Design review of the part built by this model. Coordinates are the model's own, in mm. Face numbers are marked on the shaded views. A direction names the side the tool comes from. Give positions to 0.01 mm unless a question says otherwise; leave off trailing zeros. Loops run counter-clockwise (first coordinate to the right, second up) from the corner with the lowest first, then second, coordinate; pieces in that order, holes last. Notation, with made-up numbers: (36.25, -8.75) -> (46.25, -8.75) arc R34 cw to (46.25, 22.25) -> close; hole circle Ø2 at (-34.5, 31.25). An arc over 180 degrees is marked (long way). Answer in a Markdown table with one row per item. Add a question column.
(1) Draft analysis for pull direction Z (two halves, no side actions). For the marked faces 1, 2 and 3, state which applies: +Z half, -Z half, draft (parallel to the pull), parting line (faces both ways), or undercut.
(2) Consider section A-A on y = 23.5. Write out the cut boundary in (x, z).
(3) Consider section C-C on x = 81. Write out the cut boundary in (y, z).
(4) For the marked faces 4, 5, 6 and 7, list the 3-axis set-ups (+Z, -Z, +X, -X, +Y, -Y) from which the entire face can be reached by the end or side of a thin tool; tool diameter is ignored.
(5) Consider section D-D on y = -4. Count the separate pieces of the cut face and the enclosed holes in it, then the cut area to 3 significant figures.
(6) For line 1 (Z direction, x = 46, y = 7.5); line 2 (X direction, y = 10.5, z = 29); line 3 (Z direction, x = 17, y = 26), list the stretches that pass through material, from the lowest coordinate up.
(7) Consider section B-B on x = 42. Write out the cut boundary in (y, z), then the cut area to 3 significant figures.
(8) For pin 1 (4.5 mm diameter, centred on x = 47, z = 26.5, fed in from +Y); pin 2 (5 mm diameter, centred on x = 32.5, z = 31.5, fed in from +Y); pin 3 (3.5 mm diameter, centred on y = -8.5, z = 35.5, fed in from +X), all flat-tipped, find the tip position at first contact; note any pin that passes through.
from build123d import *

# Parameters (mm, degrees)
BOSS_EXTRU_1_DEPTH       = 84
ESQUISSE6_W              = 27
ESQUISSE6_H              = 47
BOSS_EXTRU_3_DEPTH       = 17
ESQUISSE7_W              = 23.3
ESQUISSE7_H              = 14.3
ENL_V_MAT_EXTRU_4_DEPTH  = 43.3
ESQUISSE8_R              = 1.85
BOSS_EXTRU_4_DEPTH       = 3.5
ESQUISSE12_R             = 11.25
ENL_V_MAT_EXTRU_7_DEPTH  = 2.75
ESQUISSE13_W             = 27
ESQUISSE13_H             = 10
BOSS_EXTRU_5_DEPTH       = 15
ESQUISSE15_W             = 27
ESQUISSE15_H             = 15
ENL_V_MAT_EXTRU_9_DEPTH  = 4
ESQUISSE14_R             = 1.11
ENL_V_MAT_EXTRU_8_DEPTH  = 15
CONG_6_R                 = 5
CONG_7_R                 = 5
CONG_1_R                 = 10
CONG_2_R                 = 10
CONG_3_R                 = 10
CONG_4_R                 = 5
CONG_8_R                 = 5
BOSS_EXTRU_6_DEPTH       = 7.5
ESQUISSE17_R             = 2.25
ENL_V_MAT_EXTRU_10_DEPTH = 110.832109883
ESQUISSE20_W             = 91
ESQUISSE20_H             = 72.5
BOSS_EXTRU_7_DEPTH       = 7.5
ESQUISSE21_R             = 1.7
ESQUISSE21_R_2           = 1.699999999
ENL_V_MAT_EXTRU_11_DEPTH = 5
CONG_9_R                 = 5


with BuildPart() as part:
    # Esquisse1 → Boss.-Extru.1 (new body)
    with BuildSketch(Plane(origin=(0, 0, 0), x_dir=(0, 0, -1), z_dir=(1, 0, 0))):
        Polygon((-15.842295968, 13.667406166), (-15.842295968, -28.832593834), (26.657704032, -28.832593834), (26.657704032, 13.667406166), (26.657704032, 36.167406166), (30.407704032, 36.167406166), (30.407704032, 13.667406166), (30.407704032, -36.332593834), (-19.592295968, -36.332593834), (-19.592295968, 13.667406166), (-19.592295968, 36.167406166), (-15.842295968, 36.167406166), align=None)
    extrude(amount=BOSS_EXTRU_1_DEPTH)

    # Esquisse6 → Boss.-Extru.3 (add)
    with BuildSketch(Plane.XY.offset(19.592295968)):
        with Locations((42, -12.832593834)):
            Rectangle(ESQUISSE6_W, ESQUISSE6_H)
    extrude(amount=BOSS_EXTRU_3_DEPTH)

    # Esquisse7 → Enlèv. mat.-Extru.4 (cut)
    with BuildSketch(Plane(origin=(0, 10.667406166, 0), x_dir=(1, 0, 0), z_dir=(0, 1, 0))):
        with Locations((42, -26.742295968)):
            Rectangle(ESQUISSE7_W, ESQUISSE7_H)
    extrude(amount=-ENL_V_MAT_EXTRU_4_DEPTH, mode=Mode.SUBTRACT)

    # Esquisse8 → Boss.-Extru.4 (add)
    with BuildSketch(Plane(origin=(84, 0, 0), x_dir=(0, 0, -1), z_dir=(1, 0, 0))):
        with BuildLine():
            Line((-19.592295968, -36.332593834), (30.407704032, -36.332593834))
            Line((30.407704032, -36.332593834), (30.407704032, 13.667406166))
            Line((30.407704032, 13.667406166), (30.407704032, 36.167406166))
            Line((30.407704032, 36.167406166), (8.407704032, 36.167406166))
            Line((8.407704032, 36.167406166), (8.407704032, 13.667406166))
            Line((8.407704032, 13.667406166), (8.407704032, -7.582593834))
            ThreePointArc((8.407704032, -7.582593834), (5.407704032, -10.582593834), (2.407704032, -7.582593834))
            Line((2.407704032, -7.582593834), (2.407704032, 13.667406166))
            Line((2.407704032, 13.667406166), (2.407704032, 36.167406166))
            Line((2.407704032, 36.167406166), (-19.592295968, 36.167406166))
            Line((-19.592295968, 36.167406166), (-19.592295968, 13.667406166))
            Line((-19.592295968, 13.667406166), (-19.592295968, -36.332593834))
        make_face()
        with Locations((-10.167295968, 7.992406166)):
            Circle(ESQUISSE8_R, mode=Mode.SUBTRACT)
        with Locations((20.982704032, 7.992406166)):
            Circle(ESQUISSE8_R, mode=Mode.SUBTRACT)
        with Locations((20.982704032, -23.157593834)):
            Circle(ESQUISSE8_R, mode=Mode.SUBTRACT)
        with Locations((-10.167295968, -23.157593834)):
            Circle(ESQUISSE8_R, mode=Mode.SUBTRACT)
    boss_extru_4 = extrude(amount=BOSS_EXTRU_4_DEPTH)

    # Esquisse12 → Enlèv. mat.-Extru.7 (cut)
    with BuildSketch(Plane.ZY.offset(-84)):
        with Locations((-5.407704032, -7.582593834)):
            Circle(ESQUISSE12_R)
    enl_v_mat_extru_7 = extrude(amount=-ENL_V_MAT_EXTRU_7_DEPTH, mode=Mode.SUBTRACT)

    # Symétrie1: Boss.-Extru.4, Enlèv. mat.-Extru.7 across plane
    add(boss_extru_4.mirror(Plane.ZY.offset(-42)))
    add(enl_v_mat_extru_7.mirror(Plane.ZY.offset(-42)), mode=Mode.SUBTRACT)

    # Esquisse13 → Boss.-Extru.5 (add)
    with BuildSketch(Plane.XY.offset(36.592295968)):
        with Locations((42, -31.332593834)):
            Rectangle(ESQUISSE13_W, ESQUISSE13_H)
    extrude(amount=BOSS_EXTRU_5_DEPTH)

    # Esquisse15 → Enlèv. mat.-Extru.9 (cut)
    with BuildSketch(Plane.XZ.offset(36.332593834)):
        with Locations((42, 44.092295968)):
            Rectangle(ESQUISSE15_W, ESQUISSE15_H)
    extrude(amount=-ENL_V_MAT_EXTRU_9_DEPTH, mode=Mode.SUBTRACT)

    # Esquisse14 → Enlèv. mat.-Extru.8 (cut)
    with BuildSketch(Plane.XZ.offset(36.332593834)):
        with Locations(Location((35.25, 44.092295968, 0), (0, 0, 270))):
            Circle(ESQUISSE14_R)
        with Locations(Location((48.75, 44.092295968, 0), (0, 0, 270))):
            Circle(ESQUISSE14_R)
    extrude(amount=-ENL_V_MAT_EXTRU_8_DEPTH, mode=Mode.SUBTRACT)

    # Congé6
    # the kernel refuses this fillet: 5 mm, written as the material it takes off along each edge
    with BuildSketch(Plane(origin=(67.747448714, -36.332593834, 36.592295968), x_dir=(0, 0, -1), z_dir=(-1, 0, 0))) as cong_6_piece_1:
        with BuildLine():
            CenterArc((4.898979486, -5), CONG_6_R, 90, 78.463040967)
            Line((0, -4), (-0.09797959, -3.98))
            ThreePointArc((-0.09797959, -3.98), (-0.1, -2), (-0.1, 0))
            Line((-0.1, 0), (0, 0.1))
            Line((0, 0.1), (4.898979486, 0.1))
            Line((4.898979486, 0.1), (4.898979486, 0))
        make_face()
    extrude(amount=51.494897428, mode=Mode.SUBTRACT)

    # Congé7
    cong_7_edges = [part.edges().sort_by_distance(p)[0] for p in [
        (42, -32.332593834, 36.592295968),
    ]]
    fillet(cong_7_edges, radius=CONG_7_R)

    # Congé1
    cong_1_edges = [part.edges().sort_by_distance(p)[0] for p in [
        (28.5, -29.332593834, 51.592295968),
        (55.5, -29.332593834, 51.592295968),
    ]]
    fillet(cong_1_edges, radius=CONG_1_R)

    # Congé2
    cong_2_edges = [part.edges().sort_by_distance(p)[0] for p in [
        (-1.75, 36.167406166, -8.407704032),
        (-1.75, 36.167406166, -2.407704032),
        (85.75, 36.167406166, -2.407704032),
        (85.75, 36.167406166, -8.407704032),
    ]]
    fillet(cong_2_edges, radius=CONG_2_R)

    # Congé3
    cong_3_edges = [part.edges().sort_by_distance(p)[0] for p in [
        (28.5, -12.832593834, 19.592295968),
        (55.5, -12.832593834, 19.592295968),
    ]]
    fillet(cong_3_edges, radius=CONG_3_R)

    # Congé4
    cong_4_edges = [part.edges().sort_by_distance(p)[0] for p in [
        (-3.5, -0.082593834, 19.592295968),
        (87.5, -0.082593834, 19.592295968),
    ]]
    fillet(cong_4_edges, radius=CONG_4_R)

    # Congé8
    cong_8_edges = [part.edges().sort_by_distance(p)[0] for p in [
        (55.5, -7.832593834, 36.592295968),
        (28.5, -7.832593834, 36.592295968),
    ]]
    fillet(cong_8_edges, radius=CONG_8_R)

    # Esquisse16 → Boss.-Extru.6 (add)
    with BuildSketch(Plane(origin=(0, 36.167406166, 0), x_dir=(1, 0, 0), z_dir=(0, 1, 0))):
        Polygon((39.5, -15.842295968), (44.5, -15.842295968), (45.75, -15.842295968), (45.75, -19.592295968), (44.5, -19.592295968), (39.5, -19.592295968), (38.25, -19.592295968), (38.25, -15.842295968), align=None)
        Polygon((39.5, 26.657704032), (38.25, 26.657704032), (38.25, 30.407704032), (39.5, 30.407704032), (44.5, 30.407704032), (45.75, 30.407704032), (45.75, 26.657704032), (44.5, 26.657704032), align=None)
    extrude(amount=BOSS_EXTRU_6_DEPTH)

    # Esquisse17 → Enlèv. mat.-Extru.10 (cut, through all)
    with BuildSketch(Plane.XY.offset(19.592295968)):
        with Locations((42, 40.167406166)):
            Circle(ESQUISSE17_R)
    extrude(amount=-ENL_V_MAT_EXTRU_10_DEPTH, mode=Mode.SUBTRACT)

    # Esquisse20 → Boss.-Extru.7 (add)
    with BuildSketch(Plane(origin=(0, 0, -30.407704032), x_dir=(-1, 0, 0), z_dir=(0, 0, -1))):
        with Locations((-42, -0.082593834)):
            Rectangle(ESQUISSE20_W, ESQUISSE20_H)
    extrude(amount=BOSS_EXTRU_7_DEPTH)

    # Esquisse21 → Enlèv. mat.-Extru.11 (cut)
    with BuildSketch(Plane(origin=(0, 0, -37.907704032), x_dir=(-1, 0, 0), z_dir=(0, 0, -1))):
        with Locations((-75.947901314, -27.418139831)):
            Circle(ESQUISSE21_R)
        with Locations((-9.667901314, -27.162593831)):
            Circle(ESQUISSE21_R_2)
        with Locations((-75.947901314, 27.257406166)):
            Circle(ESQUISSE21_R)
    extrude(amount=-ENL_V_MAT_EXTRU_11_DEPTH, mode=Mode.SUBTRACT)

    # Congé9
    cong_9_edges = [part.edges().sort_by_distance(p)[0] for p in [
        (87.5, -0.082593834, -37.907704032),
        (-3.5, -0.082593834, -37.907704032),
    ]]
    fillet(cong_9_edges, radius=CONG_9_R)


solid = part.part
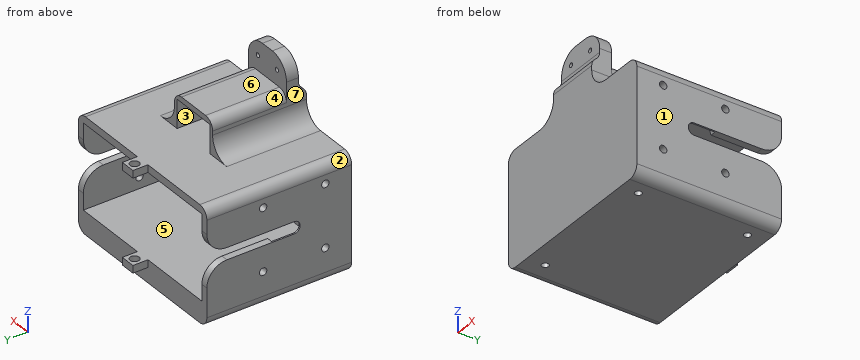
Values follow:
| question | item | result |
|---|---|---|
| 1 | face 1 | draft |
| 1 | face 2 | +Z half |
| 1 | face 3 | undercut |
| 2 | outline | (-3.5, -32.91) arc R5 ccw to (1.5, -37.91) -> (82.5, -37.91) arc R5 ccw to (87.5, -32.91) -> (87.5, -8.41) -> (84, -8.41) -> (84, -26.66) -> (0, -26.66) -> (0, -8.41) -> (-3.5, -8.41) -> close; (-3.5, -2.41) -> (0, -2.41) -> (0, 15.84) -> (84, 15.84) -> (84, -2.41) -> (87.5, -2.41) -> (87.5, 14.59) arc R5 ccw to (82.5, 19.59) -> (1.5, 19.59) arc R5 ccw to (-3.5, 14.59) -> close |
| 3 | outline | (-36.33, -37.91) -> (36.17, -37.91) -> (36.17, -26.66) -> (-28.83, -26.66) -> (-28.83, 15.84) -> (36.17, 15.84) -> (36.17, 19.59) -> (-36.33, 19.59) -> close |
| 4 | face 4 | +Z, -X, +Y |
| 4 | face 5 | +Y |
| 4 | face 6 | +Z, +X, -X, +Y |
| 4 | face 7 | +Z, -X, +Y, -Y |
| 5 | separate pieces | 2 |
| 5 | enclosed holes | 1 |
| 5 | area | 1,670 mm2 |
| 6 | line 1 | -37.91 to -26.66, 15.84 to 19.59, 33.89 to 36.59 |
| 6 | line 2 | 28.48 to 30.35, 53.65 to 55.52 |
| 6 | line 3 | -37.91 to -26.66, 15.84 to 19.59 |
| 7 | outline | (-36.33, -37.91) -> (36.17, -37.91) -> (36.17, -30.41) -> (37.92, -30.41) -> (37.92, -26.66) -> (-28.83, -26.66) -> (-28.83, 15.84) -> (37.92, 15.84) -> (37.92, 19.59) -> (-32.63, 19.59) -> (-32.63, 33.89) -> (10.67, 33.89) -> (10.67, 36.59) -> (-26.33, 36.59) -> (-26.33, 51.59) -> (-32.33, 51.59) -> (-32.33, 39.69) arc R5 cw to (-34.33, 35.69) arc R5 ccw to (-36.33, 31.69) -> close; (42.42, -30.41) -> (43.67, -30.41) -> (43.67, -26.66) -> (42.42, -26.66) -> close; (42.42, 15.84) -> (43.67, 15.84) -> (43.67, 19.59) -> (42.42, 19.59) -> close |
| 7 | area | 1,690 mm2 |
| 8 | pin 1 | y = -32.63 |
| 8 | pin 2 | y = 10.67 |
| 8 | pin 3 | x = 55.01 |
